Verification items for the finished model (mm, model axes). Give positions to 0.01 mm unless a question says otherwise; leave off trailing zeros. Write each loop counter-clockwise with the first axis right and the second up, starting at its lowest first coordinate (ties: lowest second). Pieces come first, ordered by that corner, then holes. Notation, with made-up numbers: (46.25, 27.25) -> (61.25, 27.25) arc R29 ccw to (61.25, 47.25) -> close; hole circle Ø8 at (17.5, 39.5). An arc over 180 degrees is marked (long way). Answer as CSV lines item,"result". Start each with the question number.
1) Gauge pin test, flat ends, axial feed: pin 1 Ø3.5 at (x, y) = (-10, 50) entering from +Z; pin 2 Ø1 at (x, z) = (8, 1) entering from -Y. Record the tip position at first contact, or that the pin passes through.
2) Sectioned sample at B-B on z = 1.8. Give the number of separate pieces and of enclosed holes in the cut face, and give its area (3 significant figures).
3) Material ranges on L1, parallel to Y at x = -10, z = 2.75; L2, parallel to X at y = 32, z = 2.8; L3, parallel to X at y = 49, z = 1.85, recorded low to high.
4) Sectioned sample at D-D on y = 12. Record the cut outline in (x, z), and give its area (3 significant figures).
5) Mould release check, pull along X, two halves, no side actions. Record for faces 1 (the flat face through (0, 80, 2)), 2 (the flat face through (20, 39, 2)), 3 (the cylindrical face through (11.28, 47.53, 2.03)): released by +X, released by -X, zero draft, split by the parting line, or undercut.
6) Sectioned sample at A-A on y = 70. Record the cut outline in (x, z).
7) Sectioned sample at C-C on x = -10. Record the cut outline in (y, z), and give its area (3 significant figures).
```python
from build123d import *

# Parameters (mm, degrees)
SKETCH1_W           = 40
SKETCH1_H           = 80
SKETCH1_R           = 2.78
BOSS_EXTRUDE1_DEPTH = 4


with BuildPart() as part:
    # Sketch1 → Boss-Extrude1 (new body)
    with BuildSketch(Plane.XY.offset(4)):
        with Locations((0, 40)):
            Rectangle(SKETCH1_W, SKETCH1_H)
        with Locations((-10, 70)):
            Circle(SKETCH1_R, mode=Mode.SUBTRACT)
        with Locations((-10, 50)):
            Circle(SKETCH1_R, mode=Mode.SUBTRACT)
        with Locations((-10, 30)):
            Circle(SKETCH1_R, mode=Mode.SUBTRACT)
        with Locations((-10, 10)):
            Circle(SKETCH1_R, mode=Mode.SUBTRACT)
        with Locations((10, 70)):
            Circle(SKETCH1_R, mode=Mode.SUBTRACT)
        with Locations((10, 50)):
            Circle(SKETCH1_R, mode=Mode.SUBTRACT)
        with Locations((10, 30)):
            Circle(SKETCH1_R, mode=Mode.SUBTRACT)
        with Locations((10, 10)):
            Circle(SKETCH1_R, mode=Mode.SUBTRACT)
    extrude(amount=-BOSS_EXTRUDE1_DEPTH)


solid = part.part
```
Ans:
1,pin 1,"passes through"
1,pin 2,"stops at y = 0"
2,separate pieces,"1"
2,enclosed holes,"8"
2,area,"3,010 mm²"
3,L1,"y = 0 to 7.22, 12.78 to 27.22, 32.78 to 47.22, 52.78 to 67.22, 72.78 to 80"
3,L2,"x = -20 to -11.93, -8.07 to 8.07, 11.93 to 20"
3,L3,"x = -20 to -12.59, -7.41 to 7.41, 12.59 to 20"
4,outline,"(-20, 0) -> (-11.93, 0) -> (-11.93, 4) -> (-20, 4) -> close; (-8.07, 0) -> (8.07, 0) -> (8.07, 4) -> (-8.07, 4) -> close; (11.93, 0) -> (20, 0) -> (20, 4) -> (11.93, 4) -> close"
4,area,"129 mm²"
5,face 1,"zero draft"
5,face 2,"released by +X"
5,face 3,"undercut"
6,outline,"(-20, 0) -> (-12.78, 0) -> (-12.78, 4) -> (-20, 4) -> close; (-7.22, 0) -> (7.22, 0) -> (7.22, 4) -> (-7.22, 4) -> close; (12.78, 0) -> (20, 0) -> (20, 4) -> (12.78, 4) -> close"
7,outline,"(0, 0) -> (7.22, 0) -> (7.22, 4) -> (0, 4) -> close; (12.78, 0) -> (27.22, 0) -> (27.22, 4) -> (12.78, 4) -> close; (32.78, 0) -> (47.22, 0) -> (47.22, 4) -> (32.78, 4) -> close; (52.78, 0) -> (67.22, 0) -> (67.22, 4) -> (52.78, 4) -> close; (72.78, 0) -> (80, 0) -> (80, 4) -> (72.78, 4) -> close"
7,area,"231 mm²"
